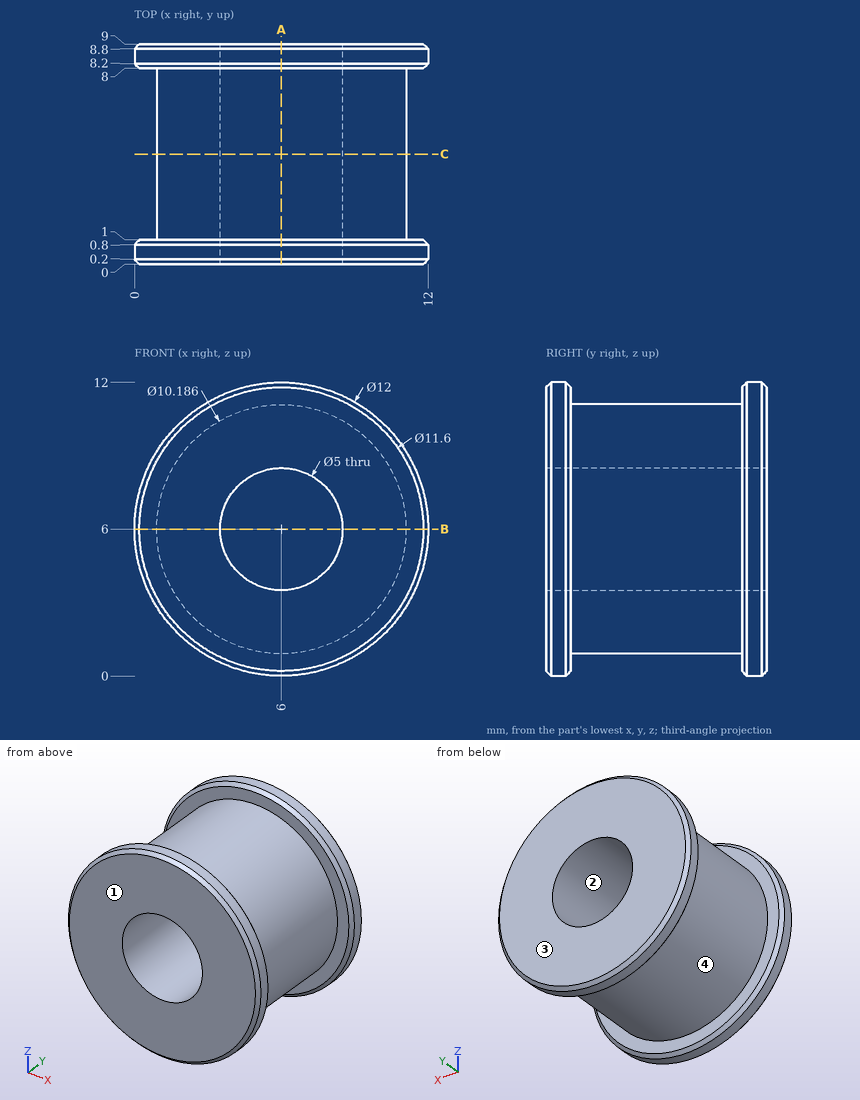
Input: dimensioned drawing with shaded views. Units: mm. Origin: part minimum x, y, z. Coordinates: 2 decimals unless noted, no trailing zeros. Loops run counter-clockwise (first coordinate to the right, second up) from the corner with the lowest first, then second, coordinate; pieces in that order, holes last. Notation, with made-up numbers: M -22.5,38 L 12.5,38 A19 ccw 12.5,55 Z; hole C 71,58.5 d11. An arc over 180 degrees is marked long. Use a Markdown table: item, result. Add a question column.
Q1. Material intervals for L1, parallel to Z at x = 6, y = 2.5; L2, parallel to Y at x = 3, z = 1.5, sorted ascending.
Q2. Section query B-B, the plane z = 6. Return loops of the section in (x, y).
Q3. Draft query along Y for the marked faces 1, 2, 3 and 4. Return one class per face: pulls with the +Y half, pulls with the -Y half, needs draft (parallel to the pull), parting line crosses it, or undercut.
Q4. Section query C-C, the plane y = 4.5. Return loops of the section in (x, z).
Q5. First-contact query: pin 1 (3 mm diameter, centred on x = 6, z = 6, fed in from -Y); pin 2 (4 mm diameter, centred on x = 8.5, y = 6.5, fed in from -Z); pin 3 (5 mm diameter, centred on x = 9.5, y = 3, fed in from -Z); pin 4 (1 mm diameter, centred on x = 10, y = 1, fed in from +Z). Flat tips, straight axial feed; report the tip coordinate or a pass-through.
Q6. Section query A-A, the plane x = 6. Return loops of the section in (y, z).
Result:
| question | item | result |
|---|---|---|
| 1 | L1 | z = 0.91 to 3.5, 8.5 to 11.09 |
| 1 | L2 | y = 0 to 1, 8 to 9 |
| 2 | outline | M 0,0.2 L 0.2,0 L 3.5,0 L 3.5,9 L 0.2,9 L 0,8.8 L 0,8.2 L 0.2,8 L 0.91,8 L 0.91,1 L 0.2,1 L 0,0.8 Z; M 8.5,0 L 11.8,0 L 12,0.2 L 12,0.8 L 11.8,1 L 11.09,1 L 11.09,8 L 11.8,8 L 12,8.2 L 12,8.8 L 11.8,9 L 8.5,9 Z |
| 3 | face 1 | pulls with the -Y half |
| 3 | face 2 | needs draft |
| 3 | face 3 | pulls with the +Y half |
| 3 | face 4 | undercut |
| 4 | outline | C 6,6 d10.19; hole C 6,6 d5 |
| 5 | pin 1 | passes through |
| 5 | pin 2 | stops at z = 0.18 |
| 5 | pin 3 | stops at z = 0.46 |
| 5 | pin 4 | stops at z = 10.84 |
| 6 | outline | M 0,0.2 L 0.2,0 L 0.8,0 L 1,0.2 L 1,0.91 L 8,0.91 L 8,0.2 L 8.2,0 L 8.8,0 L 9,0.2 L 9,3.5 L 0,3.5 Z; M 0,8.5 L 9,8.5 L 9,11.8 L 8.8,12 L 8.2,12 L 8,11.8 L 8,11.09 L 1,11.09 L 1,11.8 L 0.8,12 L 0.2,12 L 0,11.8 Z |
